The listing builds one solid part. Answer for the finished solid, in the listing's coordinates (mm). Face numbers are marked on the shaded views. A direction names the side the tool comes from. Coordinates: 2 decimals unless noted, no trailing zeros. Loops run counter-clockwise (first coordinate to the right, second up) from the corner with the lowest first, then second, coordinate; pieces in that order, holes last. Notation, with made-up numbers: (-13, 51) - (34, 51) arc R23 cw to (34, 79) - close; hole circle Ø10 at (-36, -23). An arc over 180 degrees is marked (long way). Return JSON: item names as keys, results as strings. Group by question number.
1. Section B-B (x = -6) is taken. State how many separate pieces and enclosed holes the cut face has, and give its area (3 significant figures).
2. Find the intervals of material crossed by line 1 along Y through (x, z) = (-15, 4.5); line 2 along X through (y, z) = (-48, 0.75); line 3 along Y through (x, z) = (-17, 7.5), in increasing order.
3. Section A-A (y = -27.5) is taken. Write down the section's boundary in (x, z).
4. Which of the six approach directions +Z, -Z, +X, -X, +Y, -Y give full straight-line access (tool end or side, diameter ignored) to the marked faces 1 and 2?
```python
from build123d import *

# Parameters (mm, degrees)
BOSS_EXTRUDE1_DEPTH = 10
CUT_EXTRUDE3_DEPTH  = 10


with BuildPart() as part:
    # Sketch1 → Boss-Extrude1 (new body)
    with BuildSketch(Plane.XY):
        with BuildLine():
            Line((-50, 60), (50, 60))
            ThreePointArc((50, 60), (57.071067812, 57.071067812), (60, 50))
            Line((60, 50), (60, -50))
            ThreePointArc((60, -50), (57.071067812, -57.071067812), (50, -60))
            Line((50, -60), (-50, -60))
            ThreePointArc((-50, -60), (-57.071067812, -57.071067812), (-60, -50))
            Line((-60, -50), (-60, 50))
            ThreePointArc((-60, 50), (-57.071067812, 57.071067812), (-50, 60))
        make_face()
    extrude(amount=BOSS_EXTRUDE1_DEPTH)

    # Sketch2 → Cut-Extrude3 (cut)
    with BuildSketch(Plane.XY.offset(10)):
        with BuildLine():
            Line((-8.5, 15), (-26, 15))
            add(Edge.make_bspline(
                [(-26, 15), (-25.924420184, 16.323782417), (-25.776741761, 18.910373782), (-25.18931432, 22.667480561), (-24.40218171, 26.217533319), (-23.351648748, 29.548113585), (-22.031585343, 32.658011133), (-20.475960128, 35.557827774), (-18.645030413, 38.232295908), (-16.577764404, 40.66851774), (-14.30925859, 42.854074827), (-11.88660938, 44.791927043), (-9.27275909, 46.390993922), (-6.515464901, 47.70687792), (-3.615196326, 48.758208087), (-0.544512267, 49.461107381), (2.66999963, 49.937117669), (4.870593326, 49.978770479), (5.9921875, 50)],
                knots=[0, 0, 0, 0, 1.199038563, 2.342849363, 3.436047546, 4.486744587, 5.497670872, 6.488682221, 7.459191391, 8.424610317, 9.374430501, 10.305433194, 11.225809216, 12.140057399, 13.06607119, 14.010487599, 14.985989317, 16, 16, 16, 16], degree=3))
            add(Edge.make_bspline(
                [(5.9921875, 50), (7.368928437, 49.957042053), (10.056649381, 49.873178074), (13.962121102, 49.157790502), (17.609404678, 47.961194237), (20.995848876, 46.289233684), (24.092624303, 44.165183063), (26.899217428, 41.632600324), (29.3307524, 38.638350552), (31.402645865, 35.307019593), (33.124141711, 31.779608953), (34.330494291, 28.132120076), (35.123416859, 24.461342527), (35.207986958, 21.989626722), (35.25, 20.76171875)],
                knots=[0, 0, 0, 0, 1.075374347, 2.099382735, 3.09057751, 4.06680945, 5.040638231, 6.016817125, 7.011024321, 8.044445721, 9.0776792, 10.070479129, 11.0414456, 12, 12, 12, 12], degree=3))
            add(Edge.make_bspline(
                [(35.25, 20.76171875), (35.23364234, 20.018993224), (35.200718412, 18.524070203), (34.971793962, 16.261884765), (34.628362052, 13.957584415), (34.110550426, 11.613144874), (33.464796878, 9.227908959), (32.681404487, 6.794738479), (31.742201696, 4.327428619), (30.662861893, 1.798210228), (29.375206772, -0.801128076), (27.875911369, -3.509551386), (26.125180985, -6.324657117), (24.144162236, -9.262340273), (21.923233789, -12.317967673), (19.451553804, -15.482334813), (16.757590231, -18.766591913), (14.845608498, -20.961933477), (13.86328125, -22.08984375)],
                knots=[0, 0, 0, 0, 0.728284026, 1.46585585, 2.227944881, 3.01186502, 3.81876927, 4.650621989, 5.517437689, 6.406905708, 7.346299482, 8.360816762, 9.441613733, 10.596154504, 11.834900912, 13.145207542, 14.533280747, 16, 16, 16, 16], degree=3))
            Line((13.86328125, -22.08984375), (3.6875, -33.75))
            Line((3.6875, -33.75), (36.5, -33.75))
            Line((36.5, -33.75), (36.5, -50))
            Line((36.5, -50), (-28.5, -50))
            Line((-28.5, -50), (-28.5, -41.1328125))
            Line((-28.5, -41.1328125), (0.3671875, -10.41015625))
            add(Edge.make_bspline(
                [(0.3671875, -10.41015625), (1.20296676, -9.513966827), (2.821623334, -7.778313684), (5.124804826, -5.229322392), (7.208980625, -2.810390499), (9.03093365, -0.495761262), (10.686277651, 1.639488168), (12.101200969, 3.659716873), (13.288649043, 5.546661257), (14.577792347, 7.821986632), (15.802054714, 10.535717034), (16.925389532, 13.662045728), (17.61013984, 16.650095948), (17.704657037, 18.597173702), (17.75, 19.53125)],
                knots=[0, 0, 0, 0, 1.246127091, 2.413378631, 3.493388633, 4.492180848, 5.408488754, 6.240484944, 6.999099869, 7.674939598, 8.898438119, 10.020720584, 11.050475521, 12, 12, 12, 12], degree=3))
            add(Edge.make_bspline(
                [(17.75, 19.53125), (17.716098162, 20.434896755), (17.650407917, 22.185857222), (16.928525346, 24.676589164), (15.810159831, 26.931692678), (14.234224873, 28.883782729), (12.325274062, 30.487944566), (10.119302085, 31.681075072), (7.634294101, 32.369505905), (5.892256158, 32.45567285), (4.99609375, 32.5)],
                knots=[0, 0, 0, 0, 1.062038974, 2.057870785, 3.028805853, 4.01125022, 4.991535629, 5.949134679, 6.94496649, 8, 8, 8, 8], degree=3))
            add(Edge.make_bspline(
                [(4.99609375, 32.5), (4.533124834, 32.48362502), (3.621696175, 32.451388241), (2.281967285, 32.23679673), (1.007118995, 31.858601591), (-0.217038468, 31.351873335), (-1.377440572, 30.680201393), (-2.471160416, 29.852258715), (-3.50972172, 28.889085204), (-4.488361226, 27.793692576), (-5.379050933, 26.571234082), (-6.170158274, 25.23287438), (-6.824272345, 23.77944423), (-7.400178148, 22.230131129), (-7.84434426, 20.568294193), (-8.167752291, 18.803879329), (-8.413617819, 16.93975701), (-8.470682125, 15.658348204), (-8.5, 15)],
                knots=[0, 0, 0, 0, 0.903469896, 1.778625579, 2.63899355, 3.493148037, 4.358286772, 5.247621495, 6.164656832, 7.118446693, 8.109501108, 9.111810964, 10.146451449, 11.215617525, 12.33435995, 13.498009769, 14.714554818, 16, 16, 16, 16], degree=3))
        make_face()
    extrude(amount=-CUT_EXTRUDE3_DEPTH, mode=Mode.SUBTRACT)


solid = part.part
```
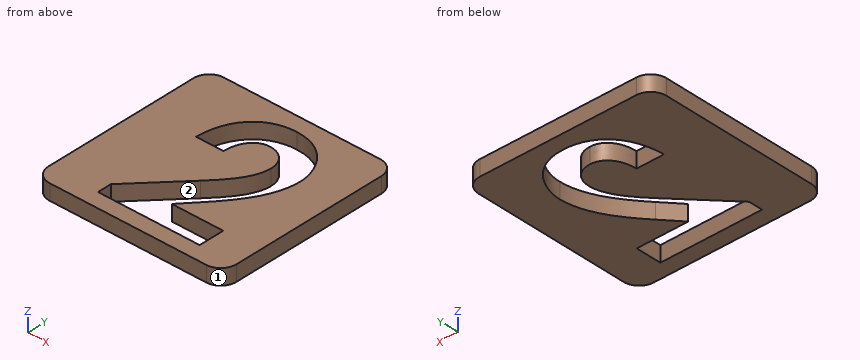
The answers:
{
 "1": {"separate pieces": "3", "enclosed holes": "0", "area": "648 mm2"},
 "2": {"line 1": "y = -60 to -50, -26.77 to 15, 42.16 to 60", "line 2": "x = -60 to -28.5, 36.5 to 60", "line 3": "y = -60 to -50, -28.89 to 15, 40.13 to 60"},
 "3": {"outline": "(-60, 0) - (-15.69, 0) - (-15.69, 10) - (-60, 10) - close; (9.14, 0) - (60, 0) - (60, 10) - (9.14, 10) - close"},
 "4": {"face 1": "+Z, -Z, +X, -Y", "face 2": "+Z, -Z"}
}
